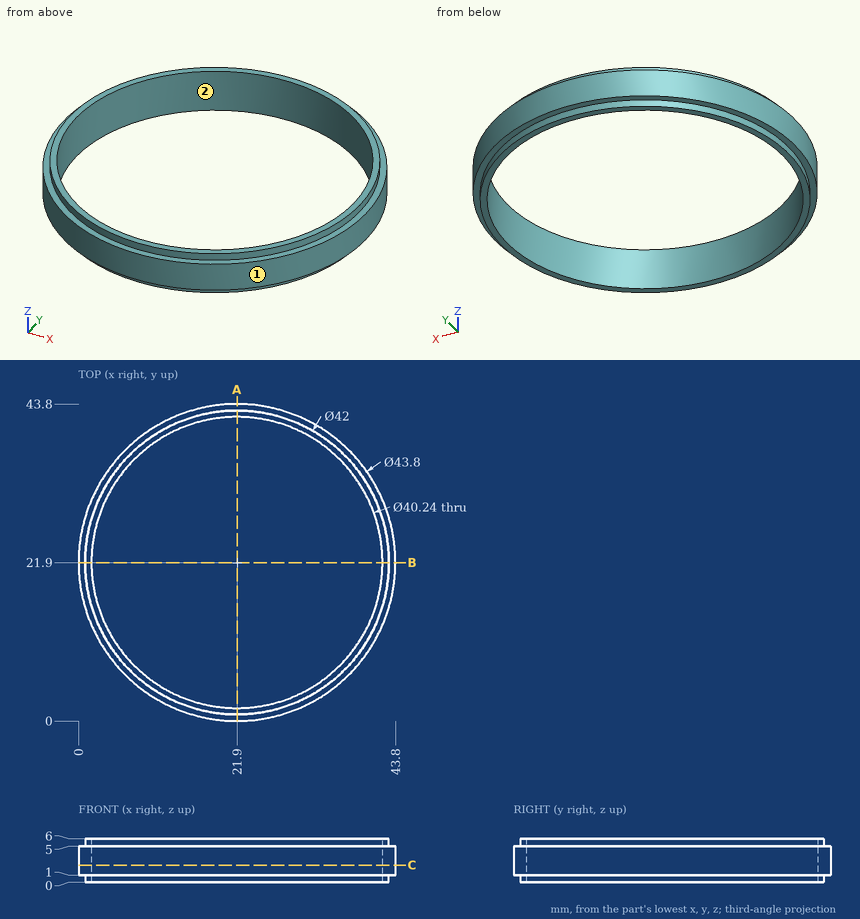
The figure shows three views and two pictorial views of one solid part (mm, origin at its lowest corner). Answer the questions. Give positions to 0.01 mm unless a question says otherwise; leave off trailing zeros. Loops run counter-clockwise (first coordinate to the right, second up) from the corner with the lowest first, then second, coordinate; pieces in that order, holes last. Notation, with made-up numbers: (57.25, 52) -> (84.25, 52) arc R21 cw to (84.25, 56) -> close; hole circle Ø7 at (-11, 26). An arc over 180 degrees is marked (long way). Use a Markdown table: item, result. Add a question column.
1. Flat-ended cylindrical pins translate along their axes: pin 1 Ø1 at (y, z) = (30.5, 2.5) entering from +X; pin 2 Ø1.5 at (x, z) = (5.5, 3) entering from -Y; pin 3 Ø1 at (x, z) = (5.5, 5) entering from +Y. Find the tip coordinate at first contact, or state that the pin passes through.
2. Determine the mould class of the marked faces 1 and 2 for opening direction X: released by +X, released by -X, zero draft, split by the parting line, or undercut.
3. Section C-C on z = 2.4 is taken. Determine the outline of the cut face in (x, y).
4. Section A-A on x = 21.9 is taken. Determine the outline of the cut face in (y, z), and give its area (3 significant figures).
5. Find the intervals of material crossed by probe 1 along Y at (x, z) = (21.9, 4.5); probe 2 along X at (y, z) = (16, 0.3); probe 3 along Z at (x, y) = (9, 4.5), in increasing order.
Results below:
| question | item | result |
|---|---|---|
| 1 | pin 1 | stops at x = 42.25 |
| 1 | pin 2 | stops at y = 6.58 |
| 1 | pin 3 | stops at y = 36.96 |
| 2 | face 1 | split by the parting line |
| 2 | face 2 | undercut |
| 3 | outline | circle Ø43.8 at (21.9, 21.9); hole circle Ø40.24 at (21.9, 21.9) |
| 4 | outline | (0, 1) -> (0.9, 1) -> (0.9, 0) -> (1.78, 0) -> (1.78, 6) -> (0.9, 6) -> (0.9, 5) -> (0, 5) -> close; (42.02, 0) -> (42.9, 0) -> (42.9, 1) -> (43.8, 1) -> (43.8, 5) -> (42.9, 5) -> (42.9, 6) -> (42.02, 6) -> close |
| 4 | area | 17.8 mm^2 |
| 5 | probe 1 | y = 0 to 1.78, 42.02 to 43.8 |
| 5 | probe 2 | x = 1.75 to 2.66, 41.14 to 42.05 |
| 5 | probe 3 | z = 1 to 5 |
